Work out the finished part from the listing and answer in its coordinate system (mm). A direction names the side the tool comes from. Give positions to 0.01 mm unless a question says otherwise; leave off trailing zeros. Loops run counter-clockwise (first coordinate to the right, second up) from the corner with the lowest first, then second, coordinate; pieces in that order, holes last. Notation, with made-up numbers: (64.25, 0) -> (105.25, 0) arc R15 ccw to (105.25, 29) -> close; hole circle Ø8 at (-17, 34). An arc over 180 degrees is marked (long way). Answer as CSV lines item,"result". Start each with the question number.
1. Find section B-B, the plane z = 2. Give the vertices of the cut face in (x, y), and give its area (3 significant figures).
2. Find the intervals of material crossed by line 1 along X through (y, z) = (1, 2.5); line 2 along X through (y, z) = (-0.5, 3.5); line 3 along Y through (x, z) = (1.5, 1), in increasing order.
3. A tool of negligible diameter and unlimited length cuts with its end or side. For faces 1 (the face through (46, 0, 0)), 2 (the face through (79.642, 0, 3)), from which of +Z, -Z, +X, -X, +Y, -Y can it reach the whole face along a straight path? Write none if from no direction.
4. Determine the mould class of faces 3 (the face through (76.467, 0, 3)), 4 (the face through (46, -4.637, 3)), 5 (the face through (0, -1.588, 3)), 6 (the face through (95.39, 0.1, 3.13)) for opening direction Y: +Y half, -Y half, draft (parallel to the pull), parting line (faces both ways), or undercut.
5. Flat-ended cylindrical pins translate along their axes: pin 1 Ø3 at (x, y) = (65.35, 0) entering from -Z; pin 2 Ø3 at (y, z) = (3, 3) entering from -X. Find the tip coordinate at first contact, or state that the pin passes through.
6. Find section C-C, the plane y = 3.75. Give the vertices of the cut face in (x, z).
7. Find section A-A, the plane y = 0. Give the vertices of the cut face in (x, z).
from build123d import *

# Parameters (mm, degrees)
SKETCH1_R           = 2.54
SKETCH1_W           = 3.175
SKETCH1_H           = 3.175
BOSS_EXTRUDE1_DEPTH = 6.35


with BuildPart() as part:
    # Sketch1 → Boss-Extrude1 (new body)
    with BuildSketch(Plane.XY):
        with BuildLine():
            Line((0, 4.636775303), (90.7542, 4.636775303))
            ThreePointArc((90.7542, 4.636775303), (95.390975303, 0), (90.7542, -4.636775303))
            Line((90.7542, -4.636775303), (0, -4.636775303))
            ThreePointArc((0, -4.636775303), (-4.636775303, 0), (0, 4.636775303))
        make_face()
        with Locations((90.7542, 0)):
            Circle(SKETCH1_R, mode=Mode.SUBTRACT)
        with Locations((65.3542, 0)):
            Circle(SKETCH1_R, mode=Mode.SUBTRACT)
        with Locations((78.0542, 0)):
            Rectangle(SKETCH1_W, SKETCH1_H, mode=Mode.SUBTRACT)
        Rectangle(SKETCH1_W, SKETCH1_H, mode=Mode.SUBTRACT)
    extrude(amount=BOSS_EXTRUDE1_DEPTH)


solid = part.part
Resolved:
1,outline,"(0, -4.64) -> (90.75, -4.64) arc R4.64 ccw to (90.75, 4.64) -> (0, 4.64) arc R4.64 ccw to start; hole (-1.59, -1.59) -> (1.59, -1.59) -> (1.59, 1.59) -> (-1.59, 1.59) -> close; hole circle Ø5.08 at (65.35, 0); hole (76.47, -1.59) -> (79.64, -1.59) -> (79.64, 1.59) -> (76.47, 1.59) -> close; hole circle Ø5.08 at (90.75, 0)"
1,area,"848 mm^2"
2,line 1,"x = -4.53 to -1.59, 1.59 to 63.02, 67.69 to 76.47, 79.64 to 88.42, 93.09 to 95.28"
2,line 2,"x = -4.61 to -1.59, 1.59 to 62.86, 67.84 to 76.47, 79.64 to 88.26, 93.24 to 95.36"
2,line 3,"y = -4.64 to -1.59, 1.59 to 4.64"
3,face 1,"-Z, +X, -X, +Y, -Y"
3,face 2,"+Z, -Z"
4,face 3,"undercut"
4,face 4,"-Y half"
4,face 5,"undercut"
4,face 6,"parting line"
5,pin 1,"passes through"
5,pin 2,"stops at x = -4.39"
6,outline,"(-2.73, 0) -> (93.48, 0) -> (93.48, 6.35) -> (-2.73, 6.35) -> close"
7,outline,"(-4.64, 0) -> (-1.59, 0) -> (-1.59, 6.35) -> (-4.64, 6.35) -> close; (1.59, 0) -> (62.81, 0) -> (62.81, 6.35) -> (1.59, 6.35) -> close; (67.89, 0) -> (76.47, 0) -> (76.47, 6.35) -> (67.89, 6.35) -> close; (79.64, 0) -> (88.21, 0) -> (88.21, 6.35) -> (79.64, 6.35) -> close; (93.29, 0) -> (95.39, 0) -> (95.39, 6.35) -> (93.29, 6.35) -> close"
